The listing builds one solid part. Answer for the finished solid, in the listing's coordinates (mm). Face numbers are marked on the shaded views. A direction names the side the tool comes from. Give positions to 0.01 mm unless a question says otherwise; leave off trailing zeros. Loops run counter-clockwise (first coordinate to the right, second up) from the corner with the lowest first, then second, coordinate; pieces in that order, holes last. Notation, with made-up numbers: M -31.5,-30 L -12.5,-30 A22 cw -12.5,7 Z; hole C -1.75,87 d2. An arc over 180 degrees is marked long. One line per item, written item: value. Start each with the question number.
Q1. Consider L1, parallel to Y at x = 11, z = -2; L2, parallel to X at y = -27.5, z = 4; L3, parallel to X at y = -34.35, z = 0. Determine where each line is inside the solid, lowest interval first.
Q2. A flat-ended cylindrical pin translates along its axis: pin 1 (6 mm diameter, centred on y = 19.5, z = -2, fed in from +X). Find the tip coordinate at first contact, or state that the pin passes through.
Q3. For the marked faces 1 and 2, determine the directions among +Z, -Z, +X, -X, +Y, -Y from which every point of the face is accessible in a straight line to the end or side of a thin tool.
Q4. A cutting plane is placed at D-D, the plane z = -3.75. Determine the outline of the cut face in (x, y), and give its area (3 significant figures).
Q5. A cutting plane is placed at A-A, the plane y = 2.5. Determine the outline of the cut face in (x, z), and give its area (3 significant figures).
Q6. A cutting plane is placed at C-C, the plane z = 0. Determine the outline of the cut face in (x, y).
Q7. A cutting plane is placed at B-B, the plane x = 21.5. Determine the outline of the cut face in (y, z), and give its area (3 significant figures).
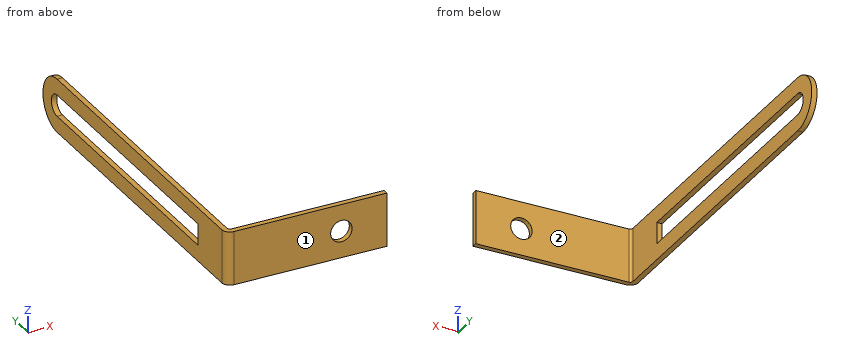
from build123d import *

# Parameters (mm, degrees)
AUFSATZ_LINEAR_AUSTRAGEN1_DEPTH = 1
AUFSATZ_LINEAR_AUSTRAGEN2_DEPTH = 10
SKIZZE3_R                       = 2
SCHNITT_LINEAR_AUSTRAGEN1_DEPTH = 72.763500472


with BuildPart() as part:
    # Skizze1 → Aufsatz-Linear austragen1 (new body)
    with BuildSketch(Plane(origin=(0, 0, 0), x_dir=(0, 0, -1), z_dir=(1, 0, 0))):
        with BuildLine():
            Line((-5, -25), (-5, -33.5))
            Line((-5, -33.5), (5, -33.5))
            Line((5, -33.5), (5, -25))
            Line((5, -25), (5, 25))
            ThreePointArc((5, 25), (0, 30), (-5, 25))
            Line((-5, 25), (-5, -25))
        make_face()
        with BuildLine():
            Line((-2, 25), (-2, -25))
            Line((-2, -25), (2, -25))
            Line((2, -25), (2, 25))
            ThreePointArc((2, 25), (0, 27), (-2, 25))
        make_face(mode=Mode.SUBTRACT)
    extrude(amount=AUFSATZ_LINEAR_AUSTRAGEN1_DEPTH)

    # Skizze2 → Aufsatz-Linear austragen2 (add)
    with BuildSketch(Plane.XY.offset(5)):
        with BuildLine():
            Line((1.5, -34), (30, -34))
            Line((30, -34), (30, -35))
            Line((30, -35), (1.5, -35))
            ThreePointArc((1.5, -35), (0.439339828, -34.560660172), (0, -33.5))
            Line((0, -33.5), (1, -33.5))
            ThreePointArc((1, -33.5), (1.146446609, -33.853553391), (1.5, -34))
        make_face()
    extrude(amount=-AUFSATZ_LINEAR_AUSTRAGEN2_DEPTH)

    # Skizze3 → Schnitt-Linear austragen1 (cut, through all)
    with BuildSketch(Plane.XZ.offset(35)):
        with Locations(Location((21.5, 0, 0), (0, 0, 270))):
            Circle(SKIZZE3_R)
    extrude(amount=-SCHNITT_LINEAR_AUSTRAGEN1_DEPTH, mode=Mode.SUBTRACT)


solid = part.part
Answer block:
1. L1: -35 to -34
1. L2: 0 to 1
1. L3: 0.26 to 19.5, 23.5 to 30
2. pin 1: x = 1
3. face 1: +Z, -Z, +X, -X, -Y
3. face 2: +Z, -Z, +X, +Y
4. outline: M 0,-33.5 A1.5 ccw 1.5,-35 L 30,-35 L 30,-34 L 1.5,-34 A0.5 cw 1,-33.5 L 1,28.31 L 0,28.31 Z
4. area: 91.9 mm^2
5. outline: M 0,-5 L 1,-5 L 1,-2 L 0,-2 Z; M 0,2 L 1,2 L 1,5 L 0,5 Z
5. area: 6.00 mm^2
6. outline: M 0,-33.5 A1.5 ccw 1.5,-35 L 19.5,-35 L 19.5,-34 L 1.5,-34 A0.5 cw 1,-33.5 L 1,-25 L 0,-25 Z; M 0,27 L 1,27 L 1,30 L 0,30 Z; M 23.5,-35 L 30,-35 L 30,-34 L 23.5,-34 Z
7. outline: M -35,-5 L -34,-5 L -34,-2 L -35,-2 Z; M -35,2 L -34,2 L -34,5 L -35,5 Z
7. area: 6.00 mm^2
